Source: CAD feature listing. Evaluate the final solid. Frame: model axes, mm. A direction names the side the tool comes from. Give positions to 0.01 mm unless a question says otherwise; leave off trailing zeros. Loops run counter-clockwise (first coordinate to the right, second up) from the corner with the lowest first, then second, coordinate; pieces in that order, holes last. Notation, with made-up numbers: (6, 20) - (62, 20) arc R18 cw to (62, 38) - close; hole circle Ø5 at (71, 59). An arc over 180 degrees is marked (long way). Put each result on its own line as item: value.
```python
from build123d import *

# Parameters (mm, degrees)
SKETCH_1_R      = 38
EXTRUDE_1_DEPTH = 17.5
SKETCH_2_R      = 6
SKETCH_2_R_2    = 3
EXTRUDE_2_DEPTH = 4
FILLET_1_R      = 6


with BuildPart() as part:
    # 草图1 → 凸台-拉伸1 (new, symmetric)
    with BuildSketch(Plane(origin=(0, 0, 0), x_dir=(1, 0, 0), z_dir=(0, 1, 0))):
        with Locations(Location((0, 0, 0), (0, 0, 270))):
            Circle(SKETCH_1_R)
    extrude(amount=EXTRUDE_1_DEPTH, both=True)

    # 草图2 → 凸台-拉伸2 (add)
    with BuildSketch(Plane(origin=(0, 17.5, 0), x_dir=(1, 0, 0), z_dir=(0, 1, 0))):
        with Locations(Location((0, 0, 0), (0, 0, 270))):
            Circle(SKETCH_2_R)
        with Locations(Location((0, 0, 0), (0, 0, 270))):
            Circle(SKETCH_2_R_2, mode=Mode.SUBTRACT)
    extrude(amount=EXTRUDE_2_DEPTH)

    # 圆角1
    fillet_1_edges = [part.edges().sort_by_distance(p)[0] for p in [
        (0, -17.5, -38),
        (0, 17.5, -38),
    ]]
    fillet(fillet_1_edges, radius=FILLET_1_R)


solid = part.part
```
1) Material intervals for line 1 along X through (y, z) = (19, 0); line 2 along Y through (x, z) = (-2.5, 11); line 3 along X through (y, z) = (1.5, -1), sorted ascending. Write a range as [from, to].
Check result:
line 1: [-6, -3], [3, 6]
line 2: [-17.5, 17.5]
line 3: [-37.99, 37.99]
2) Section query A-A, the plane x = 0. Output: boundary loops of the cut face in (y, z).
Check result:
outline: (-17.5, -32) arc R6 ccw to (-11.5, -38) - (11.5, -38) arc R6 ccw to (17.5, -32) - (17.5, -6) - (21.5, -6) - (21.5, -3) - (17.5, -3) - (17.5, 3) - (21.5, 3) - (21.5, 6) - (17.5, 6) - (17.5, 32) arc R6 ccw to (11.5, 38) - (-11.5, 38) arc R6 ccw to (-17.5, 32) - close
3) Access query for faces 1 (the cylindrical face through (1.802, 19.472, 5.723)), 2 (the flat face through (3, 21.5, 1)). Directions: +Z, -Z, +X, -X, +Y, -Y. A direction counts if a zero-diameter tool reaches every point of the face in a straight line with its end or side. Return the directions, or none.
Check result:
face 1: +Y
face 2: +Z, -Z, +X, -X, +Y
4) Section query C-C, the plane y = -10.5. Output: boundary loops of the cut face in (x, z), plus the area to 3 significant figures.
Check result:
outline: circle Ø76 at (0, 0)
area: 4,540 mm²
5) Section query B-B, the plane z = 0. Output: boundary loops of the cut face in (x, y).
Check result:
outline: (-38, -11.5) arc R6 ccw to (-32, -17.5) - (32, -17.5) arc R6 ccw to (38, -11.5) - (38, 11.5) arc R6 ccw to (32, 17.5) - (6, 17.5) - (6, 21.5) - (3, 21.5) - (3, 17.5) - (-3, 17.5) - (-3, 21.5) - (-6, 21.5) - (-6, 17.5) - (-32, 17.5) arc R6 ccw to (-38, 11.5) - close
6) Pin query (flat end, axial travel): P1, Ø4, axis at x = -18.5, y = -0.5, coming from the +Z side; P2, Ø8, axis at y = 3.5, z = -20.5, coming from the -X side; P3, Ø10, axis at y = 17, z = 25.5, coming from the +X side. Return the tip coordinate at first contact, or that it passes through.
Check result:
P1: z = 34.23
P2: x = -34.23
P3: x = 30.67
7) Mould query, pull axis X, two halves, no side actions, for faces 3 (the flat face through (0, -17.5, 0)), 4 (the cylindrical face through (-23.122, 0.161, -30.156)), 5 (the flat face through (0, 17.5, 0)), 6 (the cylindrical face through (0.9, 19.47, 2.86)). Classes: pulls with the +X half, pulls with the -X half, needs draft (parallel to the pull), parting line crosses it, or undercut.
Check result:
face 3: needs draft
face 4: parting line crosses it
face 5: undercut
face 6: undercut
